```python
from build123d import *

# Parameters (mm, degrees)
F1_DEPTH = 2.54
F3_DEPTH = 2.54


with BuildPart() as f1:
    # F0 (on Top) → F1 (new body)
    with BuildSketch(Plane.XY):
        with BuildLine():
            Line((0, 6.029797), (0, 2.854797))
            ThreePointArc((0, 2.854797), (1.281656, 2.941419), (2.54, 3.199709))
            ThreePointArc((2.54, 3.199709), (9.525, 12.379797), (2.54, 21.559886))
            ThreePointArc((2.54, 21.559886), (1.281656, 21.818175), (0, 21.904797))
            Line((0, 21.904797), (0, 18.729797))
            ThreePointArc((0, 18.729797), (6.35, 12.379797), (0, 6.029797))
        make_face()
        with BuildLine():
            ThreePointArc((2.54, 3.199709), (1.281656, 2.941419), (0, 2.854797))
            Line((0, 2.854797), (0, 0.314797))
            Line((0, 0.314797), (2.54, 0.314797))
            Line((2.54, 0.314797), (2.54, 3.199709))
        make_face()
        with BuildLine():
            ThreePointArc((0, 21.904797), (1.281656, 21.818175), (2.54, 21.559886))
            Line((2.54, 21.559886), (2.54, 24.444797))
            Line((2.54, 24.444797), (0, 24.444797))
            Line((0, 24.444797), (0, 21.904797))
        make_face()
    extrude(amount=F1_DEPTH)

    # F2 (on face) → F3 (join)
    with BuildSketch(Plane.XY.offset(2.54)):
        with BuildLine():
            Line((0, 6.029797), (0, 4.442297))
            ThreePointArc((0, 4.442297), (7.9375, 12.379797), (0, 20.317297))
            Line((0, 20.317297), (0, 18.729797))
            ThreePointArc((0, 18.729797), (6.35, 12.379797), (0, 6.029797))
        make_face()
    extrude(amount=F3_DEPTH)


solid = f1.part
```
Source: CAD feature listing. Evaluate the final solid. Frame: model axes, mm. A direction names the side the tool comes from. Coordinates: 2 decimals unless noted, no trailing zeros. Write each loop counter-clockwise with the first axis right and the second up, starting at its lowest first coordinate (ties: lowest second). Pieces come first, ordered by that corner, then holes. Notation, with made-up numbers: (33.25, -11.75) -> (71.25, -11.75) arc R29 ccw to (71.25, 9.25) -> close; hole circle Ø10 at (21.25, 8). An arc over 180 degrees is marked (long way). Return JSON: item names as keys, results as strings. Group by question number.
1) Contact query for flat-ended pins moving along their axis: P1, Ø5, axis at x = 4, y = 10, coming from the +Z side; P2, Ø2, axis at y = 2, z = 1, coming from the +X side; P3, Ø4, axis at x = 8.5, y = 6.5, coming from the +Z side. Output: stop coordinate, or through.
2) Section query B-B, the plane z = 2.1. Return loops of the section in (x, y) (3 decimals).
3) Section query A-A, the plane x = 3. Return loops of the section in (y, z).
4) Section query C-C, the plane x = 7.25. Return loops of the section in (y, z), plus the area to 3 significant figures.
5) Ray query, line 1 along Z through (x, y) = (2, 4); line 2 along Y through (x, z) = (1, 3.1); line 3 along Y through (x, z) = (5.75, 3.6). Return the intervals inside material, ascending.
6) Set-up query: faces 5 (the face through (8, 11, 2.54)), 6 (the face through (2.54, 23, 1)), 7 (the face through (0, 4, 2)), 8 (the face through (2.54, 2, 1)). Return all of +Z, -Z, +X, -X, +Y, -Y with unobstructed straight access to the full face (end or side cutting, diameter ignored); none if empty.
7) Section query D-D, the plane y = 2.5. Return loops of the section in (x, z), plus the area to 3 significant figures.
8) Mould query, pull axis Y, two halves, no side actions, for faces 1 (the face through (1, 24.445, 1)), 2 (the face through (0, 21, 2)), 3 (the face through (9.523, 12.206, 1.252)), 4 (the face through (6.35, 12.52, 2.5)). Classes: +Y half, -Y half, draft (parallel to the pull), parting line (faces both ways), or undercut.
From the geometry:
{
 "1": {"P1": "z = 5.08", "P2": "x = 2.54", "P3": "z = 2.54"},
 "2": {"outline": "(0, 0.315) -> (2.54, 0.315) -> (2.54, 3.2) arc R9.525 ccw to (2.54, 21.56) -> (2.54, 24.445) -> (0, 24.445) -> (0, 18.73) arc R6.35 cw to (0, 6.03) -> close"},
 "3": {"outline": "(3.34, 0) -> (6.78, 0) -> (6.78, 5.08) -> (5.03, 5.08) -> (5.03, 2.54) -> (3.34, 2.54) -> close; (17.98, 0) -> (21.42, 0) -> (21.42, 2.54) -> (19.73, 2.54) -> (19.73, 5.08) -> (17.98, 5.08) -> close"},
 "4": {"outline": "(6.2, 0) -> (18.56, 0) -> (18.56, 2.54) -> (15.61, 2.54) -> (15.61, 5.08) -> (9.15, 5.08) -> (9.15, 2.54) -> (6.2, 2.54) -> close", "area": "47.8 mm²"},
 "5": {"line 1": "0 to 2.54", "line 2": "4.51 to 6.11, 18.65 to 20.25", "line 3": "6.91 to 9.69, 15.07 to 17.85"},
 "6": {"face 5": "+Z, +X", "face 6": "+Z, -Z, +X, +Y", "face 7": "+Z, -Z, -X, +Y, -Y", "face 8": "+Z, -Z, +X, -Y"},
 "7": {"outline": "(0, 0) -> (2.54, 0) -> (2.54, 2.54) -> (0, 2.54) -> close", "area": "6.45 mm²"},
 "8": {"face 1": "+Y half", "face 2": "draft", "face 3": "parting line", "face 4": "undercut"}
}
